Read the model definition and answer for the solid it produces. Units are mm, in the model's axes. A direction names the side the tool comes from. Give positions to 0.01 mm unless a question says otherwise; leave off trailing zeros. Loops run counter-clockwise (first coordinate to the right, second up) from the corner with the lowest first, then second, coordinate; pieces in that order, holes last. Notation, with made-up numbers: M -23,60 L 5,60 A24 ccw 5,96 Z; hole C 38.25,73 d10. An arc over 180 degrees is marked long. Return JSON: item names as keys, results as strings. Group by question number.
```python
from build123d import *

# Parameters (mm, degrees)
F0_W     = 50.8
F0_H     = 508
F1_DEPTH = 50.8
F2_W     = 25.4
F2_H     = 3.81
F3_DEPTH = 508.001
F4_W     = 3.81
F4_H     = 25.4
F5_DEPTH = 508.001
F7_DEPTH = 508.001


with BuildPart() as f1:
    # F0 (on Top) → F1 (new body)
    with BuildSketch(Plane.XY):
        with Locations((25.4, 254)):
            Rectangle(F0_W, F0_H)
    extrude(amount=F1_DEPTH)

    # F2 (on face) → F3 (cut, through all)
    with BuildSketch(Plane(origin=(0, 508, 0), x_dir=(-1, 0, 0), z_dir=(0, 1, 0))):
        with Locations((-38.1, 48.895)):
            Rectangle(F2_W, F2_H)
    extrude(amount=-F3_DEPTH, mode=Mode.SUBTRACT)

    # F4 (on face) → F5 (cut, through all)
    with BuildSketch(Plane(origin=(0, 508, 0), x_dir=(-1, 0, 0), z_dir=(0, 1, 0))):
        with Locations((-1.905, 12.7)):
            Rectangle(F4_W, F4_H)
    extrude(amount=-F5_DEPTH, mode=Mode.SUBTRACT)

    # F6 (on face) → F7 (cut, through all)
    with BuildSketch(Plane(origin=(0, 508, 0), x_dir=(-1, 0, 0), z_dir=(0, 1, 0))):
        with BuildLine():
            Line((0, 50.8), (-19.05, 50.8))
            Line((-19.05, 50.8), (-19.05, 46.99))
            ThreePointArc((-19.05, 46.99), (-8.273693, 42.526307), (-3.81, 31.75))
            Line((-3.81, 31.75), (0, 31.75))
            Line((0, 31.75), (0, 50.8))
        make_face()
    extrude(amount=-F7_DEPTH, mode=Mode.SUBTRACT)


solid = f1.part
```
1. Find section C-C (x = 46). Write down the section's boundary in (y, z), and give its area (3 significant figures).
2. Straight lines are drawn through the part: line 1 along Z through (x, y) = (30.5, 70.5); line 2 along X through (y, z) = (102, 22); line 3 along Z through (x, y) = (3.5, 487.5). For each, find the intervals that lie inside material, in ascending order.
3. Find section A-A (y = 203). Write down the section's boundary in (x, z).
4. Find section B-B (z = 19). Write down the section's boundary in (x, y).
5. Flat-ended cylindrical pins translate along their axes: P1, Ø1.1, axis at y = 162, z = 49.5, coming from the +X side; P2, Ø4, axis at x = 1.5, y = 211, coming from the +Z side; P3, Ø3, axis at y = 249, z = 49.5, coming from the -X side; P4, Ø10, axis at x = 26, y = 258, coming from the -Z side. Find the tip coordinate at first contact, or state that the pin passes through.
6. The mould has two halves that part along Y. Classify faces 3 (the flat face through (38, 258, 46.99)), 4 (the flat face through (25, 0, 25)), 5 (the flat face through (25, 508, 25)): +Y half, -Y half, draft (parallel to the pull), parting line (faces both ways), or undercut.
7. For faces 1 (the cylindrical face through (8.39, 257.56, 42.64)), 2 (the flat face through (3.81, 258, 13)), determine the directions among +Z, -Z, +X, -X, +Y, -Y from which every point of the face is accessible in a straight line to the end or side of a thin tool.
Result:
{
 "1": {"outline": "M 0,0 L 508,0 L 508,46.99 L 0,46.99 Z", "area": "23,900 mm2"},
 "2": {"line 1": "z = 0 to 46.99", "line 2": "x = 3.81 to 50.8", "line 3": "z = 25.4 to 31.75"},
 "3": {"outline": "M 0,25.4 L 3.81,25.4 L 3.81,0 L 50.8,0 L 50.8,46.99 L 25.4,46.99 L 25.4,50.8 L 19.05,50.8 L 19.05,46.99 A15.24 ccw 3.81,31.75 L 0,31.75 Z"},
 "4": {"outline": "M 3.81,0 L 50.8,0 L 50.8,508 L 3.81,508 Z"},
 "5": {"P1": "stops at x = 25.4", "P2": "stops at z = 31.75", "P3": "stops at x = 19.05", "P4": "stops at z = 0"},
 "6": {"face 3": "draft", "face 4": "-Y half", "face 5": "+Y half"},
 "7": {"face 1": "+Z, -X, +Y, -Y", "face 2": "-Z, -X, +Y, -Y"}
}
